Model file for the job. Use its own axes, mm. Face numbers are marked on the shaded views. A direction names the side the tool comes from. Round coordinates to 2 decimals unless told otherwise and drop trailing zeros. Loops run counter-clockwise (first coordinate to the right, second up) from the corner with the lowest first, then second, coordinate; pieces in that order, holes last. Notation, with made-up numbers: M -36,-34 L -16,-34 A15 ccw -16,-6 Z; hole C 9,67 d10. An arc over 180 degrees is marked long. Use a Markdown table: item, result. Add a question column.
Item 1: Wall check: L1, parallel to X at y = 0.25, z = 4.25; L2, parallel to X at y = 0, z = 1.6; L3, parallel to X at y = -1.75, z = 2.25. Give the ranges that are in metal, low to high. Write a range as from..to.
Item 2: Saw through at C-C on z = 5. Give the number of separate pieces and of enclosed holes in the cut face, then the cut area to 3 significant figures.
Item 3: Pin check, flat tips, straight feed: P1, Ø3, axis at x = 14.5, y = 1, coming from the +Z side; P2, Ø2, axis at x = -12.5, z = 2.5, coming from the +Y side; P3, Ø3.5, axis at y = 11.5, z = 3, coming from the -X side. Stop position of each tip, or through.
Item 4: Saw through at A-A on x = 4.4. Write the cut outline in (y, z).
Item 5: Two-plate mould, pull along Y, no slides. Class the marked faces 1, 2, 3 and 4: +Y half, -Y half, draft (parallel to the pull), parting line (faces both ways), or undercut.
Item 6: Saw through at B-B on y = 4.25. Write the cut outline in (x, z).
Item 7: Saw through at D-D on y = 11.5. Write the cut outline in (x, z).
Item 8: Tool access for the marked faces 5, 6, 7 and 8: list every direction of +Z, -Z, +X, -X, +Y, -Y with a clear straight run to the whole face (end or side of a thin tool).
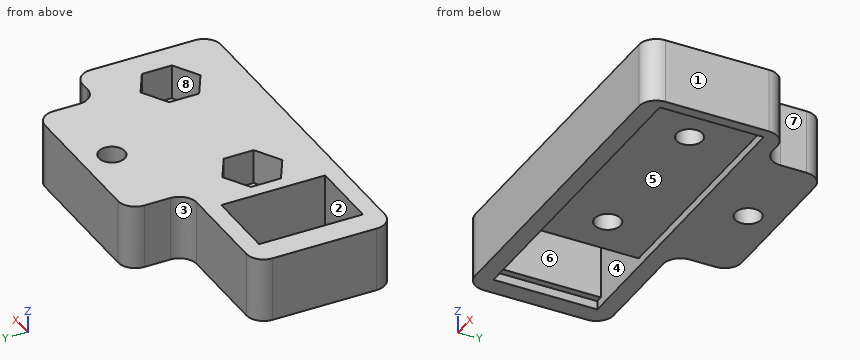
Autodesk Inventor part; units mm, degrees
ref_plane "YZ Plane" through (0, 0, 0) normal (1, 0, 0) x (0, 1, 0)
ref_plane "XZ Plane" through (0, 0, 0) normal (0, 1, 0) x (-1, 0, 0)
ref_plane "XY Plane" through (0, 0, 0) normal (0, 0, 1) x (1, 0, 0)
sketch "Sketch1" plane through (0, 0, 0) normal (0, 0, 1) x (1, 0, 0)
  line L0 (-10.2, 5) -> (-10.2, -5)
  line L1 (-10.2, -5) -> (16.5, -5)
  line L2 (16.5, -5) -> (16.5, 5)
  line L3 (16.5, 5) -> (-10.2, 5)
  circle A0 centre (13.4, 0) radius 1.5
  circle A1 centre (-4.6, 0) radius 1.5
  line L4 (-16.5, 5) -> (-16.5, -5)
  line L5 (-20.5, 8) -> (19.5, 8)
  line L6 (19.5, 8) -> (19.5, -8)
  line L7 (19.5, -8) -> (-20.5, -8)
  line L8 (-20.5, -8) -> (-20.5, 8)
  line L9 (-9.2, 8) -> (-9.2, -8)
  line L10 (-17.5, 8) -> (-17.5, -8)
  line L11 (-17.5, 6) -> (-9.2, 6)
  line L12 (-17.5, -6) -> (-9.2, -6)
  point P0 (0, 0)
  dimension "d0" = 3
  dimension "d1" = 3
  dimension "d2" = 3
  dimension "d3" = 4
  dimension "d4" = 1
  dimension "d5" = 1
  dimension "d6" = 1
  dimension "d7" = 1
extrude "Extrusion1" add sketch "Sketch1" along normal blind 7.5 contours L9 L5 L6 L7 L1 L2 L3 | L3 L2 L1 L9 | L11 L10 L5 L9 | L9 L7 L10 L12 | L10 L7 L8 L5
sketch "Sketch2" plane through (0, 0, 7.5) normal (0, 0, 1) x (1, 0, 0)
  circle A0 centre (-4.6, 0) radius 1.5
  circle A1 centre (13.4, 0) radius 1.5
  line L0 (-1.6, -1.7321) -> (-4.6, -3.4641)
  line L1 (-4.6, -3.4641) -> (-7.6, -1.7321)
  line L2 (-7.6, -1.7321) -> (-7.6, 1.7321)
  line L3 (-7.6, 1.7321) -> (-4.6, 3.4641)
  line L4 (-4.6, 3.4641) -> (-1.6, 1.7321)
  line L5 (-1.6, 1.7321) -> (-1.6, -1.7321)
  circle A2 centre (13.4, 0) radius 1.5
  line L6 (10.4, 1.7321) -> (13.4, 3.4641)
  line L7 (13.4, 3.4641) -> (16.4, 1.7321)
  line L8 (16.4, 1.7321) -> (16.4, -1.7321)
  line L9 (16.4, -1.7321) -> (13.4, -3.4641)
  line L10 (13.4, -3.4641) -> (10.4, -1.7321)
  line L11 (10.4, -1.7321) -> (10.4, 1.7321)
  point P0 (0, 0)
  dimension "d10" = 6
  dimension "d11" = 6
extrude "Extrusion2" cut sketch "Sketch2" against normal blind 4
sketch "Sketch3" plane through (-20.5, 8, 0) normal (0, 1, 0) x (1, 0, 0)
  line L0 (40, 0) -> (0, 0)
  line L1 (0, -7.5) -> (40, -7.5)
  line L2 (34.9, 0) -> (14.9, 0)
  line L3 (14.9, 0) -> (14.9, -7.5)
  line L4 (14.9, -7.5) -> (34.9, -7.5)
  line L5 (34.9, -7.5) -> (34.9, 0)
  line L6 (13.1, 5) -> (13.1, 2)
  line L7 (13.1, 2) -> (36.7, 2)
  line L8 (36.7, 2) -> (36.7, 5)
  line L9 (36.7, 5) -> (30.7, 5)
  line L10 (30.7, 5) -> (30.7, 13)
  line L11 (30.7, 13) -> (26.3, 13)
  line L12 (26.3, 13) -> (26.3, 5)
  line L13 (26.3, 5) -> (23.5, 5)
  line L14 (23.5, 5) -> (23.5, 13)
  line L15 (23.5, 13) -> (19.1, 13)
  line L16 (19.1, 13) -> (19.1, 5)
  line L17 (19.1, 5) -> (13.1, 5)
  line L18 (24.9, 15.273) -> (24.9, -16.6011) construction
  point P0 (20.5, 0)
  dimension "d14" = 20
  dimension "d15" = 2.8
  dimension "d16" = 1.4
  dimension "d17" = 10
extrude "Extrusion3" add sketch "Sketch3" along normal blind 7 contours L5 L1 L3 L0
sketch "Sketch4" plane through (0, 0, 0) normal (0, 0, -1) x (-1, 0, 0)
  circle A0 centre (-4.4, 11.5) radius 1.5
  line L0 (-19.5, 8) -> (-14.4, 8)
  line L1 (-19.5, -8) -> (-19.5, 8)
  line L2 (20.5, -8) -> (-19.5, -8)
  line L3 (20.5, 8) -> (20.5, -8)
  line L4 (5.6, 8) -> (20.5, 8)
  line L5 (5.6, 8) -> (5.6, 15)
  line L6 (-14.4, 15) -> (5.6, 15)
  line L7 (-14.4, 8) -> (-14.4, 15)
  circle A1 centre (4.6, 0) radius 1.5
  circle A2 centre (-13.4, 0) radius 1.5
  line L8 (17.5, -6) -> (17.5, 6)
  line L9 (9.2, -6) -> (17.5, -6)
  line L10 (9.2, 6) -> (9.2, -6)
  line L11 (17.5, 6) -> (9.2, 6)
  point P0 (0, 0)
  dimension "d20" = 3
  dimension "d21" = 20
  dimension "d22" = 7
  dimension "d23" = 3.5
  dimension "d24" = 10
extrude "Extrusion4" cut sketch "Sketch4" against normal through all contours A0
fillet "Fillet1" radius 2 8 edges at (-5.6, 15, 3.75) (-5.6, 8, 3.75) (-20.5, 8, 3.75) (-20.5, -8, 3.75) (19.5, -8, 3.75) (19.5, 8, 3.75) (14.4, 8, 3.75) (14.4, 15, 3.75)
sketch "Sketch5" plane through (0, 0, 0) normal (0, 0, -1) x (-1, 0, 0)
  line L0 (18.3, -6) -> (-18.3, -6)
  line L1 (-18.3, -6) -> (-18.3, 6)
  line L2 (-18.3, 6) -> (18.3, 6)
  line L3 (18.3, 6) -> (18.3, -6)
  point P0 (0, 0)
  dimension "d28" = 12
  dimension "d29" = 36.6
  dimension "d30" = 18.3
  dimension "d31" = 6
extrude "Extrusion5" cut sketch "Sketch5" against normal blind 1
equation "\"d1\" = d0"
equation "\"d2\" = d0"
equation "\"d11\" = d10"
equation "\"d16\" = 0.5 * d15"
equation "\"d17\" = 0.5 * d14"
equation "\"d23\" = 0.5 * d22"
equation "\"d24\" = 0.5 * d21"
properties part number "optical endstop base"
Entries:
| question | item | result |
|---|---|---|
| 1 | L1 | -20.5..-17.5, -9.2..-7.6, -1.6..10.4, 16.4..19.5 |
| 1 | L2 | -20.5..-17.5, -9.2..-6.1, -3.1..11.9, 14.9..19.5 |
| 1 | L3 | -20.5..-17.5, -9.2..19.5 |
| 2 | separate pieces | 1 |
| 2 | enclosed holes | 4 |
| 2 | area | 608 mm2 |
| 3 | P1 | z = 3.5 |
| 3 | P2 | y = 8 |
| 3 | P3 | x = -5.62 |
| 4 | outline | M -8,0 L -6,0 L -6,1 L 6,1 L 6,0 L 10,0 L 10,7.5 L -8,7.5 Z; M 13,0 L 15,0 L 15,7.5 L 13,7.5 Z |
| 5 | face 1 | draft |
| 5 | face 2 | undercut |
| 5 | face 3 | +Y half |
| 5 | face 4 | undercut |
| 6 | outline | M -20.5,0 L -18.3,0 L -18.3,1 L -17.5,1 L -17.5,7.5 L -20.5,7.5 Z; M -9.2,1 L 18.3,1 L 18.3,0 L 19.5,0 L 19.5,7.5 L -9.2,7.5 Z |
| 7 | outline | M -5.6,0 L 2.9,0 L 2.9,7.5 L -5.6,7.5 Z; M 5.9,0 L 14.4,0 L 14.4,7.5 L 5.9,7.5 Z |
| 8 | face 5 | -Z |
| 8 | face 6 | +Z, -Z |
| 8 | face 7 | +Z, -Z, +X, +Y |
| 8 | face 8 | +Z |
